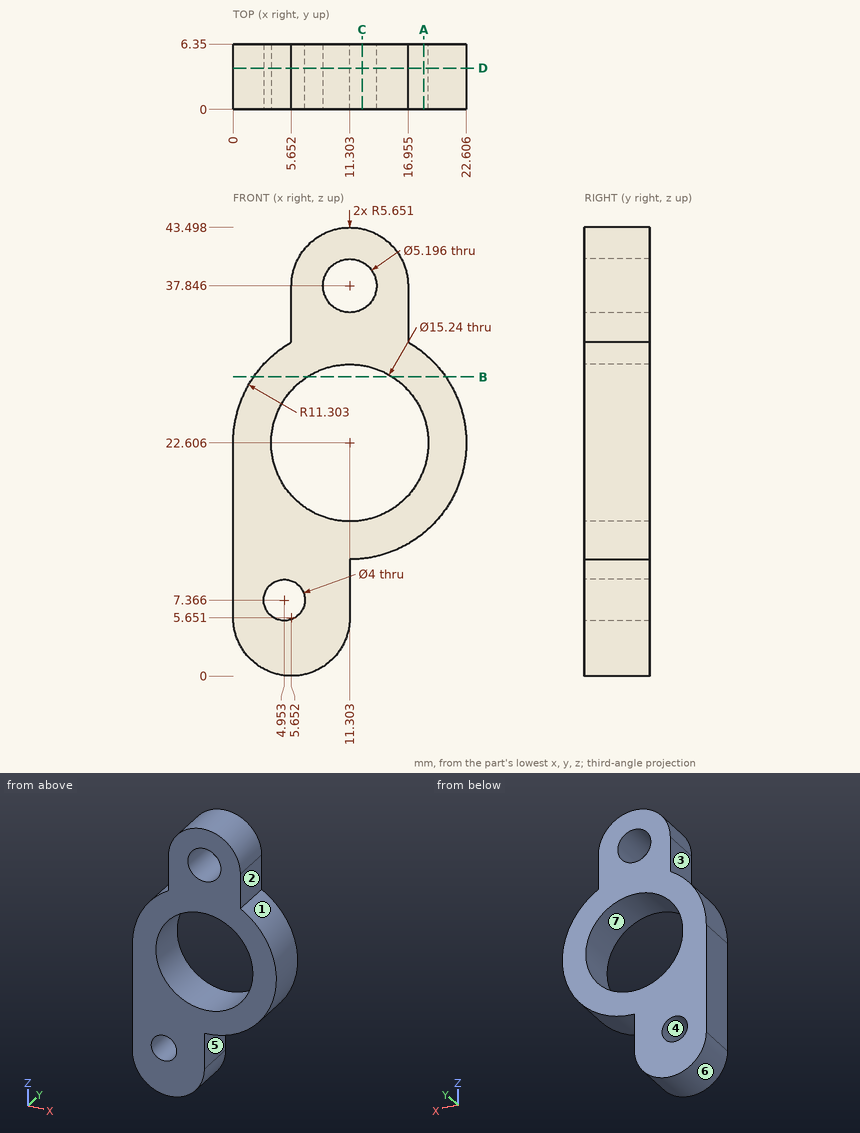
Design review of the part shown in the three views and the two pictorial views. Dimensions are in mm from the part's minimum x, y and z. A direction names the side the tool comes from. Round coordinates to 2 decimals unless told otherwise and drop trailing zeros. Write each loop counter-clockwise with the first axis right and the second up, starting at its lowest first coordinate (ties: lowest second). Pieces come first, ordered by that corner, then holes. Notation, with made-up numbers: (64.5, 85.5) - (76.5, 85.5) arc R19 ccw to (76.5, 122.5) - close; hole circle Ø8 at (-13.75, 9). An arc over 180 degrees is marked (long way). Return JSON: item names as keys, results as strings. Group by question number.
Item 1: We need section D-D on y = 4. Write out the cut boundary in (x, z) (1 decimal).
Item 2: Machinability: for the marked faces 1, 2 and 3, which of the approach directions +Z, -Z, +X, -X, +Y, -Y give a long, thin tool a straight path to every point of the face, cutting with its end or side? Answer none if there is none.
Item 3: The part is to be moulded in two halves that separate along X. For the marked faces 4, 5, 6 and 7, say which applies: pulls with the +X half, pulls with the -X half, needs draft (parallel to the pull), parting line crosses it, or undercut.
Item 4: We need section A-A on x = 18.5. Write out the cut boundary in (y, z).
Item 5: We need section C-C on x = 12.5. Write out the cut boundary in (y, z).
Item 6: Insertion check: P1, Ø1, axis at x = 18, y = 1.5, coming from the -Z side; P2, Ø2.5, axis at y = 4.5, z = 35, coming from the +X side (1 decimal); P3, Ø3, axis at y = 4.5, z = 8, coming from the +X side. Each pin has a flat end and moves straight along its axis. Give the tip position at first contact, or say it passes through.
Item 7: We need section B-B on z = 29. Write out the cut boundary in (x, y).
Item 8: For probe 1 along Z at (x, y) = (4.5, 2.25) (1 decimal); probe 2 along Z at (x, y) = (10, 6.25) (1 decimal); probe 3 along X at (y, z) = (2.5, 23.5) (1 decimal), list the stretches that pass through material, from the lowest coordinate up. Write a range as [from, to].
Model answer:
{
 "1": {"outline": "(0, 5.7) arc R5.7 ccw to (11.3, 5.7) - (11.3, 11.3) arc R11.3 ccw to (17, 32.4) - (17, 37.8) arc R5.7 ccw to (5.7, 37.8) - (5.7, 32.4) arc R11.3 ccw to (0, 22.6) - close; hole circle Ø4 at (5, 7.4); hole circle Ø15.2 at (11.3, 22.6); hole circle Ø5.2 at (11.3, 37.8)"},
 "2": {"face 1": "+X, +Y, -Y", "face 2": "+Z, +X, +Y, -Y", "face 3": "+Z, -X, +Y, -Y"},
 "3": {"face 4": "undercut", "face 5": "pulls with the +X half", "face 6": "parting line crosses it", "face 7": "undercut"},
 "4": {"outline": "(0, 13.89) - (6.35, 13.89) - (6.35, 20.1) - (0, 20.1) - close; (0, 25.11) - (6.35, 25.11) - (6.35, 31.32) - (0, 31.32) - close"},
 "5": {"outline": "(0, 11.37) - (6.35, 11.37) - (6.35, 15.08) - (0, 15.08) - close; (0, 30.13) - (6.35, 30.13) - (6.35, 35.54) - (0, 35.54) - close; (0, 40.15) - (6.35, 40.15) - (6.35, 43.37) - (0, 43.37) - close"},
 "6": {"P1": "stops at z = 13.15", "P2": "stops at x = 17", "P3": "stops at x = 11.3"},
 "7": {"outline": "(1.98, 0) - (7.16, 0) - (7.16, 6.35) - (1.98, 6.35) - close; (15.45, 0) - (20.62, 0) - (20.62, 6.35) - (15.45, 6.35) - close"},
 "8": {"probe 1": "z = [0.1, 5.4], [9.3, 19.2], [26, 31.6]", "probe 2": "z = [2, 15.1], [30.1, 35.6], [40.1, 43.3]", "probe 3": "x = [0, 3.7], [18.9, 22.6]"}
}
